from build123d import *

# Parameters (mm, degrees)
SKETCH1_R                       = 2.75
BOSS_EXTRUDE1_DEPTH             = 3
BOSS_EXTRUDE2_START             = -3
SKETCH2_W                       = 70
SKETCH2_H                       = 50
SKETCH2_R                       = 2.75
BOSS_EXTRUDE2_DEPTH             = 3
FILLET1_R                       = 5
TAP_DRILL_FOR_M4X0_7_TAP1_D     = 3.3
TAP_DRILL_FOR_M4X0_7_TAP1_DEPTH = 5
TAP_DRILL_FOR_M4X0_7_TAP1_TIP   = 0.991420021
FILLET2_R                       = 1


with BuildPart() as part:
    # Sketch1 → Boss-Extrude1 (new body)
    with BuildSketch(Plane.XY):
        with BuildLine():
            Line((-27.5, 40.954554701), (-27.5, 43.77942119))
            ThreePointArc((-27.5, 43.77942119), (-27.675848554, 44.243388065), (-28.115043604, 44.474246643))
            ThreePointArc((-28.115043604, 44.474246643), (-29.494269709, 44.515011098), (-30.857622009, 44.302415486))
            ThreePointArc((-30.857622009, 44.302415486), (-33.320623763, 43.783640888), (-35.816700763, 43.459442898))
            ThreePointArc((-35.816700763, 43.459442898), (-36.454446159, 42.968046035), (-36.279664044, 42.182144463))
            Line((-36.279664044, 42.182144463), (-34.910050506, 40.812530925))
            ThreePointArc((-34.910050506, 40.812530925), (-34.823341406, 40.37661484), (-35.192893219, 40.129688213))
            Line((-35.192893219, 40.129688213), (-38.85, 40.129688213))
            ThreePointArc((-38.85, 40.129688213), (-39.910660172, 40.569028041), (-40.35, 41.629688213))
            Line((-40.35, 41.629688213), (-40.35, 44.839311769))
            ThreePointArc((-40.35, 44.839311769), (-40.127638883, 45.755826908), (-39.51, 46.468544718))
            ThreePointArc((-39.51, 46.468544718), (-39.333648382, 46.591125418), (-39.154570787, 46.709688213))
            ThreePointArc((-39.154570787, 46.709688213), (-37.336364984, 47.543852346), (-35.356465997, 47.829688213))
            Line((-35.356465997, 47.829688213), (-34.963696275, 47.829688213))
            ThreePointArc((-34.963696275, 47.829688213), (-34.853104675, 47.781026744), (-34.81426707, 47.666614851))
            Line((-34.81426707, 47.666614851), (-34.859717037, 47.147119361))
            ThreePointArc((-34.859717037, 47.147119361), (-34.807933564, 46.994570171), (-34.660478097, 46.929688213))
            Line((-34.660478097, 46.929688213), (-33.8, 46.929688213))
            ThreePointArc((-33.8, 46.929688213), (-31.798990845, 47.174505883), (-29.916025641, 47.89451656))
            ThreePointArc((-29.916025641, 47.89451656), (-29.70812219, 48.570368729), (-30.383974359, 48.778272181))
            ThreePointArc((-30.383974359, 48.778272181), (-31.625663196, 48.261025539), (-32.941176471, 47.980383271))
            ThreePointArc((-32.941176471, 47.980383271), (-33.129888119, 47.994076587), (-33.3, 48.076911006))
            Line((-33.3, 48.076911006), (-33.5, 48.076911006))
            Line((-33.5, 48.076911006), (-33.5, 81.629688213))
            Line((-33.5, 81.629688213), (-34.6, 81.629688213))
            Line((-34.6, 81.629688213), (-34.913048957, 80.461373602))
            ThreePointArc((-34.913048957, 80.461373602), (-34.962999168, 80.340783124), (-35.042458479, 80.237229734))
            Line((-35.042458479, 80.237229734), (-36.153553391, 79.126134822))
            ThreePointArc((-36.153553391, 79.126134822), (-36.315765065, 79.017748447), (-36.507106781, 78.979688213))
            Line((-36.507106781, 78.979688213), (-37.319402422, 78.979688213))
            ThreePointArc((-37.319402422, 78.979688213), (-37.920814021, 79.072254311), (-38.466555295, 79.341384124))
            Line((-38.466555295, 79.341384124), (-39.923576436, 80.361601311))
            ThreePointArc((-39.923576436, 80.361601311), (-40.237010833, 80.719004742), (-40.35, 81.180753355))
            Line((-40.35, 81.180753355), (-40.35, 81.315474651))
            ThreePointArc((-40.35, 81.315474651), (-40.273784436, 81.698387585), (-40.05675537, 82.022932669))
            Line((-40.05675537, 82.022932669), (-34.383177792, 87.69087524))
            ThreePointArc((-34.383177792, 87.69087524), (-33.896725598, 88.01565007), (-33.323044738, 88.129688213))
            Line((-33.323044738, 88.129688213), (-27.5, 88.129688213))
            Line((-27.5, 88.129688213), (-27.5, 90.954554701))
            Line((-27.5, 90.954554701), (22.5, 90.954554701))
            Line((22.5, 90.954554701), (22.5, 40.954554701))
            Line((22.5, 40.954554701), (-27.5, 40.954554701))
        make_face()
        with Locations((-17.5, 71.3)):
            Circle(SKETCH1_R, mode=Mode.SUBTRACT)
        with Locations((17.5, 55.3)):
            Circle(SKETCH1_R, mode=Mode.SUBTRACT)
    extrude(amount=BOSS_EXTRUDE1_DEPTH)

    # Sketch2 → Boss-Extrude2 (add)
    with BuildSketch(Plane.XY.offset(3).offset(BOSS_EXTRUDE2_START)):
        with Locations((7.5, 65.954554701)):
            Rectangle(SKETCH2_W, SKETCH2_H)
        with Locations((-17.5, 71.3)):
            Circle(SKETCH2_R, mode=Mode.SUBTRACT)
        with Locations((17.5, 55.3)):
            Circle(SKETCH2_R, mode=Mode.SUBTRACT)
    extrude(amount=BOSS_EXTRUDE2_DEPTH)

    # Fillet1
    fillet1_edges = [part.edges().sort_by_distance(p)[0] for p in [
        (42.5, 40.954554701, 1.5),
        (42.5, 90.954554701, 1.5),
    ]]
    fillet(fillet1_edges, radius=FILLET1_R)

    # Tap Drill for M4x0.7 Tap1
    with Locations(Plane.XY.offset(3)):
        with Locations((37.5, 45.954554701), (37.5, 85.954554701)):
            Hole(TAP_DRILL_FOR_M4X0_7_TAP1_D / 2, depth=TAP_DRILL_FOR_M4X0_7_TAP1_DEPTH)
            with Locations((0, 0, -(TAP_DRILL_FOR_M4X0_7_TAP1_DEPTH + TAP_DRILL_FOR_M4X0_7_TAP1_TIP / 2))):  # 118° drill point
                Cone(0, TAP_DRILL_FOR_M4X0_7_TAP1_D / 2, TAP_DRILL_FOR_M4X0_7_TAP1_TIP, mode=Mode.SUBTRACT)

    # Fillet2
    fillet2_edges = [part.edges().sort_by_distance(p)[0] for p in [
        (-27.5, 90.954554701, 1.5),
        (-27.5, 40.954554701, 1.5),
        (-27.5, 88.129688213, 1.5),
    ]]
    fillet(fillet2_edges, radius=FILLET2_R)


solid = part.part
Check sheet for the modelled part. Datum: model origin and axes. Units: mm. A direction names the side the tool comes from. Give positions to 0.01 mm unless a question says otherwise; leave off trailing zeros. Loops run counter-clockwise (first coordinate to the right, second up) from the corner with the lowest first, then second, coordinate; pieces in that order, holes last. Notation, with made-up numbers: M -37.5,48 L -25.5,48 A16 ccw -25.5,60 Z; hole C -0.75,32 d3. An arc over 180 degrees is marked long. Answer as a JSON object with one key per item and string values. Group by question number.
Q1. Go/stop test with flat-tipped pins: P1, Ø0.9, axis at y = 60.5, z = 2, coming from the -X side; P2, Ø0.7, axis at y = 89.5, z = 1.5, coming from the -X side. Record where each tip stops, or that it passes through.
Q2. Cross-section at C-C on x = -6.5. Record the cut outline in (y, z), then the cut area to 3 significant figures.
Q3. Release check for a two-part mould opening along X. For faces 1 (the cylindrical face through (41.074, 42.458, 1.521)), 2 (the flat face through (-27.5, 43, 1)), 3 (the flat face through (2, 66, 0)) record: released by +X, released by -X, zero draft, split by the parting line, or undercut.
Q4. Material ranges on line 1 along Y through (x, z) = (37.5, 1.55); line 2 along Y through (x, z) = (-17.5, 1.85); line 3 along X through (y, z) = (62.5, 1.45), recorded low to high. Write a range as [from, to].
Q5. Cross-section at B-B on z = 1. Give the number of separate pieces and of enclosed holes in the cut face, then the cut area to 3 significant figures.
Q6. Access from +Z, -Z, +X, -X, +Y, -Y to the whole of each face (thin tool, end or side, straight path). Record for faces 4 (the cylindrical face through (-37.363, 47.536, 1.479)), 5 (the cylindrical face through (-33.29, 43.79, 1.48)), 6 (the flat face through (-31, 88.13, 1)), 7 (the flat face through (6, 40.955, 1)).
Q7. Cross-section at A-A on x = 17.5. Record the cut outline in (y, z).
Q8. Cross-section at D-D on x = -32. Record the cut outline in (y, z).
Evaluation:
{
 "1": {"P1": "stops at x = -33.5", "P2": "stops at x = -27.5"},
 "2": {"outline": "M 40.95,0 L 90.95,0 L 90.95,3 L 40.95,3 Z", "area": "150 mm2"},
 "3": {"face 1": "released by +X", "face 2": "undercut", "face 3": "zero draft"},
 "4": {"line 1": "y = [40.95, 44.3], [47.6, 84.3], [87.6, 90.95]", "line 2": "y = [40.95, 68.55], [74.05, 90.95]", "line 3": "x = [-33.5, 42.5]"},
 "5": {"separate pieces": "1", "enclosed holes": "4", "area": "3,760 mm2"},
 "6": {"face 4": "+Z, -Z, -X", "face 5": "+Z, -Z", "face 6": "+Z, -Z, -X, +Y", "face 7": "+Z, -Z, +X, -Y"},
 "7": {"outline": "M 40.95,0 L 52.55,0 L 52.55,3 L 40.95,3 Z; M 58.05,0 L 90.95,0 L 90.95,3 L 58.05,3 Z"},
 "8": {"outline": "M 44.04,0 L 47.13,0 L 47.13,3 L 44.04,3 Z; M 48.16,0 L 88.13,0 L 88.13,3 L 48.16,3 Z"}
}
